from build123d import *

# Parameters (mm, degrees)
SKETCH1_R           = 77.4600051
BOSS_EXTRUDE1_DEPTH = 3.175
SKETCH24_R          = 22.1615
SKETCH24_R_2        = 2.0193
SKETCH24_R_3        = 2.54
CUT_EXTRUDE14_DEPTH = 110.590991442


with BuildPart() as part:
    # Sketch1 → Boss-Extrude1 (new body)
    with BuildSketch(Plane(origin=(0, 0, 0), x_dir=(1, 0, 0), z_dir=(0, 1, 0))):
        with Locations(Location((0, 0, 0), (0, 0, 270))):
            Circle(SKETCH1_R)
    extrude(amount=BOSS_EXTRUDE1_DEPTH)

    # Sketch24 → Cut-Extrude14 (cut, through all)
    with BuildSketch(Plane(origin=(0, 3.175, 0), x_dir=(1, 0, 0), z_dir=(0, 1, 0))):
        with Locations(Location((0, 0, 0), (0, 0, 270))):
            Circle(SKETCH24_R)
        with Locations(Location((0, 33.02, 0), (0, 0, 270))):
            Circle(SKETCH24_R_2)
        with Locations(Location((33.02, 0, 0), (0, 0, 270))):
            Circle(SKETCH24_R_2)
        with Locations(Location((-33.02, 0, 0), (0, 0, 270))):
            Circle(SKETCH24_R_2)
        with Locations(Location((0, -33.02, 0), (0, 0, 270))):
            Circle(SKETCH24_R_2)
        with Locations(Location((-30.48, -30.48, 0), (0, 0, 270))):
            Circle(SKETCH24_R_3)
        with Locations(Location((-25.4, 25.4, 0), (0, 0, 270))):
            Circle(SKETCH24_R_2)
        with BuildLine():
            Line((-27.903416949, -9.657564215), (-23.915755925, -17.31778977))
            ThreePointArc((-23.915755925, -17.31778977), (-26.616171022, -25.882412255), (-35.180793507, -23.181997158))
            Line((-35.180793507, -23.181997158), (-39.16845453, -15.521771603))
            ThreePointArc((-39.16845453, -15.521771603), (-36.468039434, -6.957149118), (-27.903416949, -9.657564215))
        make_face()
    extrude(amount=-CUT_EXTRUDE14_DEPTH, mode=Mode.SUBTRACT)


solid = part.part
Geometry: final body of the model. Coordinates: model frame, mm. A direction names the side the tool comes from. Give positions to 0.01 mm unless a question says otherwise; leave off trailing zeros. Loops run counter-clockwise (first coordinate to the right, second up) from the corner with the lowest first, then second, coordinate; pieces in that order, holes last. Notation, with made-up numbers: M -14.5,3.5 L -3.5,3.5 A31 ccw -3.5,35.5 Z; hole C -37,84 d5. An arc over 180 degrees is marked long. Put each result on its own line as item: value.
1) Reachability of faces 1 (the flat face through (-25.94, 1.61, 13.43)), 2 (the flat face through (-16, 0, 16)) from +Z, -Z, +X, -X, +Y, -Y: full face, straight path, thin tool, end or side. Return the list, or none.
Computed values:
face 1: +Y, -Y
face 2: +Z, -Z, +X, -X, -Y
2) Cut plane B-B, the plane y = 2.15. Give the number of separate pieces and of enclosed holes in the cut face, plus the area to 3 significant figures.
Computed values:
separate pieces: 1
enclosed holes: 8
area: 17,000 mm^2
3) Material intervals for L1, parallel to X at y = 2.05, z = 0; L2, parallel to X at y = 2.4, z = 18; L3, parallel to X at y = 1.15, z = -25.4, sorted ascending. Write a range as from..to.
Computed values:
L1: x = -77.46..-35.04, -31..-22.16, 22.16..31, 35.04..77.46
L2: x = -75.34..-37.88, -23.61..-12.93, 12.93..75.34
L3: x = -73.18..-27.42, -23.38..73.18
4) Mould query, pull axis X, two halves, no side actions, for faces 3 (the flat face through (-16, 3.175, 16)), 4 (the cylindrical face through (-26.493, 1.61, 25.817)), 5 (the cylindrical face through (-0.773, 1.61, 34.885)), 6 (the cylindrical face through (23.27, 1.57, 73.88)). Classes: released by +X, released by -X, zero draft, split by the parting line, or undercut.
Computed values:
face 3: zero draft
face 4: undercut
face 5: undercut
face 6: split by the parting line
5) Cut plane D-D, the plane z = -25.4. Return the cut outline in (x, y) (3 decimals), plus the area to 3 significant figures.
Computed values:
outline: M -73.177,0 L -27.419,0 L -27.419,3.175 L -73.177,3.175 Z; M -23.381,0 L 73.177,0 L 73.177,3.175 L -23.381,3.175 Z
area: 452 mm^2
6) Cut plane A-A, the plane x = 0. Return the cut outline in (y, z) (1 decimal), plus the area to 4 significant figures.
Computed values:
outline: M 0,-77.5 L 3.2,-77.5 L 3.2,-35 L 0,-35 Z; M 0,-31 L 3.2,-31 L 3.2,-22.2 L 0,-22.2 Z; M 0,22.2 L 3.2,22.2 L 3.2,31 L 0,31 Z; M 0,35 L 3.2,35 L 3.2,77.5 L 0,77.5 Z
area: 325.5 mm^2
7) First-contact query: P1, Ø1.5, axis at y = 1, z = -28.5, coming from the -X side; P2, Ø3.5, axis at x = 0, z = 33.02, coming from the -Y side. Flat tips, straight axial feed; report the tip coordinate or a pass-through.
Computed values:
P1: stops at x = -72.32
P2: passes through
8) Cut plane C-C, the plane z = 0. Return the cut outline in (x, y) (1 decimal).
Computed values:
outline: M -77.5,0 L -35,0 L -35,3.2 L -77.5,3.2 Z; M -31,0 L -22.2,0 L -22.2,3.2 L -31,3.2 Z; M 22.2,0 L 31,0 L 31,3.2 L 22.2,3.2 Z; M 35,0 L 77.5,0 L 77.5,3.2 L 35,3.2 Z
